```python
from build123d import *

# Parameters (mm, degrees)
BOSS_EXTRUDE1_DEPTH = 20
SKETCH2_R           = 10
CUT_EXTRUDE1_DEPTH  = 10
CUT_EXTRUDE2_DEPTH  = 20
SKETCH4_R           = 5
CUT_EXTRUDE3_DEPTH  = 20


with BuildPart() as part:
    # Sketch1 → Boss-Extrude1 (new body)
    with BuildSketch(Plane.XY):
        with BuildLine():
            Line((46.177047915, 17.530175597), (-42.328960588, 17.530175597))
            Line((-42.328960588, 17.530175597), (-42.328960588, 43.184091105))
            ThreePointArc((-42.328960588, 43.184091105), (-62.602792244, 54.153197241), (-84.660607586, 47.459743594))
            Line((-84.660607586, 47.459743594), (-84.660607586, 27.459743594))
            ThreePointArc((-84.660607586, 27.459743594), (-112.119008023, -0.001343253), (-84.657921177, -27.45974369))
            Line((-84.657921177, -27.45974369), (-84.657921177, -47.45974369))
            ThreePointArc((-84.657921177, -47.45974369), (-63.493440882, -56.226358468), (-42.328960588, -47.45974369))
            Line((-42.328960588, -47.45974369), (-42.328960588, -21.805828182))
            Line((-42.328960588, -21.805828182), (46.177047915, -21.805828182))
            Line((46.177047915, -21.805828182), (46.177047915, 17.530175597))
        make_face()
    extrude(amount=BOSS_EXTRUDE1_DEPTH)

    # Sketch2 → Cut-Extrude1 (cut)
    with BuildSketch(Plane.XY.offset(20)):
        with Locations((29.612265592, -1.914255488)):
            Circle(SKETCH2_R)
        with Locations((-62.725631092, 38.929575976)):
            Circle(SKETCH2_R)
        with Locations((-63.794313785, -40.25113932)):
            Circle(SKETCH2_R)
    extrude(amount=-CUT_EXTRUDE1_DEPTH, mode=Mode.SUBTRACT)

    # Sketch3 → Cut-Extrude2 (cut)
    with BuildSketch(Plane.XY.offset(20)):
        with BuildLine():
            Line((-95.412007987, -10.461867625), (-95.412007987, 6.633356649))
            ThreePointArc((-95.412007987, 6.633356649), (-87.536563025, 14.508801611), (-79.661118062, 6.633356649))
            Line((-79.661118062, 6.633356649), (-79.661118062, -10.461867625))
            ThreePointArc((-79.661118062, -10.461867625), (-87.536563025, -18.337312588), (-95.412007987, -10.461867625))
        make_face()
    extrude(amount=-CUT_EXTRUDE2_DEPTH, mode=Mode.SUBTRACT)

    # Sketch4 → Cut-Extrude3 (cut)
    with BuildSketch(Plane.XY.offset(20)):
        with Locations((-62.725631092, 38.929575976)):
            Circle(SKETCH4_R)
        with Locations((-63.794313785, -40.25113932)):
            Circle(SKETCH4_R)
        with Locations((29.612265592, -1.914255488)):
            Circle(SKETCH4_R)
    extrude(amount=-CUT_EXTRUDE3_DEPTH, mode=Mode.SUBTRACT)


solid = part.part
```
Geometry: final body of the model. Coordinates: model frame, mm. A direction names the side the tool comes from. Round coordinates to 2 decimals unless told otherwise and drop trailing zeros. Order: outer loops, then holes, each group sorted by start corner. A loop starts at its lowest first (then second) coordinate and runs counter-clockwise, first axis right, second up. Notation, with made-up numbers: M -15.5,-31 L 7.5,-31 A28 cw 7.5,7 Z; hole C 43.5,13 d9. An arc over 180 degrees is marked long. Use one line per item in the form item = value. Start each with the question number.
Q1. Cut plane B-B (y = -43.5). Return loops of the section in (x, z), and give its area (3 significant figures).
Q2. Access query for faces 5 (the face through (32, 3, 10)), 6 (the face through (-42.329, 30, 10)), 7 (the face through (-79.661, -2, 10)), 8 (the face through (-42.329, -35, 10)). Directions: +Z, -Z, +X, -X, +Y, -Y. A direction counts if a zero-diameter tool reaches every point of the face in a straight line with its end or side. Return the directions, or none.
Q3. Cut plane C-C (x = -4). Return loops of the section in (y, z).
Q4. Pin query (flat end, axial travel): pin 1 Ø4 at (y, z) = (-13.5, 5) entering from -X; pin 2 Ø6 at (x, y) = (-67.5, 37) entering from +Z; pin 3 Ø5 at (x, z) = (-36, 9.5) entering from -Y; pin 4 Ø18 at (x, y) = (29.61, -1.91) entering from -Z. Return the tip coordinate at first contact, or that it passes through.
Q5. Cut plane D-D (z = 4.5). Return loops of the section in (x, y), and give its area (3 significant figures).
Q6. Material intervals for line 1 (X direction, y = -41, z = 10.75); line 2 (X direction, y = -3, z = 19); line 3 (Y direction, x = 5.5, z = 1.5), sorted ascending. Write a range as [from, to].
Q7. Cut plane A-A (y = -4). Return loops of the section in (x, z).
Q8. Mould query, pull axis X, two halves, no side actions, for faces 1 (the face through (-66.16, -35.67, 10)), 2 (the face through (46.177, -2, 10)), 3 (the face through (3, 17.53, 10)), 4 (the face through (-112.112, 0.602, 9.86)). Classes: +X half, -X half, draft (parallel to the pull), parting line (faces both ways), or undercut.
Geometry results:
q1.outline = M -84.66,0 L -67.59,0 L -67.59,10 L -73.25,10 L -73.25,20 L -84.66,20 Z; M -59.99,0 L -42.33,0 L -42.33,20 L -54.34,20 L -54.34,10 L -59.99,10 Z
q1.area = 581 mm^2
q2.face_5 = +Z
q2.face_6 = +Z, -Z, +X, +Y
q2.face_7 = +Z, -Z
q2.face_8 = +Z, -Z, +X, -Y
q3.outline = M -21.81,0 L 17.53,0 L 17.53,20 L -21.81,20 Z
q4.pin_1 = -109.59
q4.pin_2 = 10
q4.pin_3 = -21.81
q4.pin_4 = 0
q5.outline = M -84.66,-47.46 A29.93 ccw -42.33,-47.46 L -42.33,-21.81 L 46.18,-21.81 L 46.18,17.53 L -42.33,17.53 L -42.33,43.18 A29.93 ccw -84.66,47.46 L -84.66,27.46 A27.46 ccw -84.66,-27.46 Z; hole M -95.41,-10.46 A7.88 ccw -79.66,-10.46 L -79.66,6.63 A7.88 ccw -95.41,6.63 Z; hole C -63.79,-40.25 d10; hole C -62.73,38.93 d10; hole C 29.61,-1.91 d10
q5.area = 8,410 mm^2
q6.line_1 = [-84.66, -73.77], [-53.82, -42.33]
q6.line_2 = [-111.95, -95.41], [-79.66, 19.67], [39.55, 46.18]
q6.line_3 = [-21.81, 17.53]
q7.outline = M -111.83,0 L -95.41,0 L -95.41,20 L -111.83,20 Z; M -79.66,0 L 25.07,0 L 25.07,10 L 19.83,10 L 19.83,20 L -79.66,20 Z; M 34.16,0 L 46.18,0 L 46.18,20 L 39.39,20 L 39.39,10 L 34.16,10 Z
q8.face_1 = undercut
q8.face_2 = +X half
q8.face_3 = draft
q8.face_4 = -X half
